Input: part model. Units: mm. Frame: model coordinates. Face numbers are marked on the shaded views. A direction names the side the tool comes from. Coordinates: 2 decimals unless noted, no trailing zeros. Loops run counter-clockwise (first coordinate to the right, second up) from the corner with the lowest first, then second, coordinate; pieces in that order, holes last. Notation, with made-up numbers: (-23, 44) - (24, 44) arc R12 cw to (24, 54) - close; hole circle Ø5 at (15, -36). An arc over 180 degrees is marked (long way). Use a Markdown table: item, result. Add a question column.
1. Ray query, L1, parallel to X at y = -1.75, z = -1.75; L2, parallel to Z at x = 14.5, y = 1; L3, parallel to Z at x = 5.25, y = 1.75. Return the intervals inside material, ascending. Write a range as [from, to].
2. Section query A-A on x = 5.25. Return the cut outline in (y, z).
3. Contact query for a flat-ended pin moving along its axis: P1, Ø4, axis at x = 8, z = 1, coming from the -Y side. Output: stop coordinate, or through.
4. Draft query along Z for the marked faces 3, 4, 5 and 6. Return one class per face: released by +Z, released by -Z, zero draft, split by the parting line, or undercut.
5. Access query for the marked faces 1 and 2. Directions: +Z, -Z, +X, -X, +Y, -Y. A direction counts if a zero-diameter tool reaches every point of the face in a straight line with its end or side. Return the directions, or none.
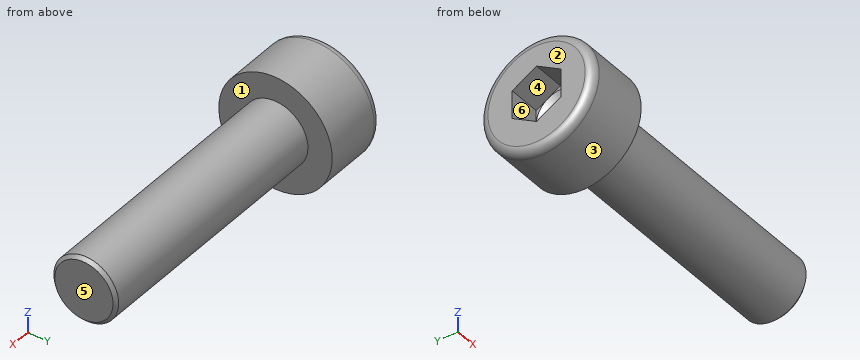
```python
from build123d import *

# Parameters (mm, degrees)
SKETCH1_R           = 3.5
BASEHEAD_DEPTH      = 4
SKETCH2_R           = 2
BASEBODY_DEPTH      = 16
HEXAGONSOCKET_DEPTH = 2
TOPFILLET_R         = 0.5
CHAMFER1_SIZE       = 0.2


with BuildPart() as part:
    # Sketch1 → BaseHead (new body)
    with BuildSketch(Plane(origin=(0, 0, 0), x_dir=(0, 0, -1), z_dir=(1, 0, 0))):
        Circle(SKETCH1_R)
    extrude(amount=BASEHEAD_DEPTH)

    # Sketch2 → BaseBody (add)
    with BuildSketch(Plane(origin=(4, 0, 0), x_dir=(0, 0, -1), z_dir=(1, 0, 0))):
        Circle(SKETCH2_R)
    extrude(amount=BASEBODY_DEPTH)

    # Sketch3 → HexagonSocket (cut)
    with BuildSketch(Plane(origin=(0, 0, 0), x_dir=(0, 0, -1), z_dir=(1, 0, 0))):
        Polygon((1.732050808, 0), (0.866025404, 1.5), (-0.866025404, 1.5), (-1.732050808, 0), (-0.866025404, -1.5), (0.866025404, -1.5), align=None)
    extrude(amount=HEXAGONSOCKET_DEPTH, mode=Mode.SUBTRACT)

    # Sketch4 → Cut-Revolve1 (revolve, cut)
    with BuildSketch(Plane(origin=(-4.19613823, 0.75, 0), x_dir=(-1, 0, 0), z_dir=(0, 0, 1))):
        Polygon((-6.19613823, 2.25), (-7.062163633, 0.75), (-6.19613823, 0.75), align=None)
    revolve(axis=Axis((0.838992387, 0, 0), (-1, 0, 0)), mode=Mode.SUBTRACT)

    # TopFillet
    topfillet_edges = [part.edges().sort_by_distance(p)[0] for p in [
        (0, 0, 3.5),
    ]]
    fillet(topfillet_edges, radius=TOPFILLET_R)

    # Chamfer1
    chamfer1_edges = [part.edges().sort_by_distance(p)[0] for p in [
        (20, 0, 2),
    ]]
    chamfer(chamfer1_edges, length=CHAMFER1_SIZE)


solid = part.part
```
Resolved:
| question | item | result |
|---|---|---|
| 1 | L1 | [0, 4] |
| 1 | L2 | [-1.73, 1.73] |
| 1 | L3 | [-0.97, 0.97] |
| 2 | outline | circle Ø4 at (0, 0) |
| 3 | P1 | y = -2 |
| 4 | face 3 | split by the parting line |
| 4 | face 4 | undercut |
| 4 | face 5 | zero draft |
| 4 | face 6 | undercut |
| 5 | face 1 | +X |
| 5 | face 2 | +Z, -Z, -X, +Y, -Y |
